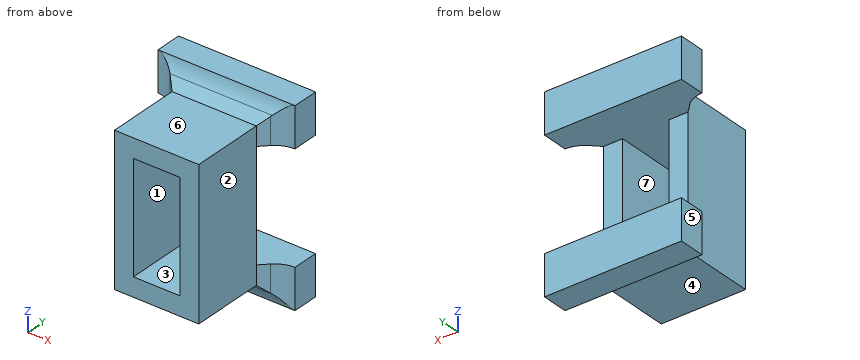
Autodesk Inventor part; units mm, degrees
ref_plane "YZ Plane" through (0, 0, 0) normal (1, 0, 0) x (0, 1, 0)
ref_plane "XZ Plane" through (0, 0, 0) normal (0, 1, 0) x (-1, 0, 0)
ref_plane "XY Plane" through (0, 0, 0) normal (0, 0, 1) x (1, 0, 0)
sketch "Sketch1" plane through (0, 0, 0) normal (0, 1, 0) x (-1, 0, 0)
  line L0 (0, 0) -> (10.16, 0)
  line L1 (10.16, 0) -> (10.16, -17.78)
  line L2 (10.16, -17.78) -> (0, -17.78)
  line L3 (0, -17.78) -> (0, 0)
  line L4 (7.874, -15.494) -> (7.874, -2.286)
  line L5 (7.874, -2.286) -> (2.286, -2.286)
  line L6 (2.286, -2.286) -> (2.286, -15.494)
  line L7 (2.286, -15.494) -> (7.874, -15.494)
  dimension "d0" = 17.78
  dimension "d1" = 10.16
  dimension "d2" = 2.286
extrude "Extrusion1" add sketch "Sketch1" along normal blind 8.89
sketch "Sketch2" plane through (0, 8.89, 0) normal (0, 1, 0) x (1, 0, 0)
  line L0 (-10.16, 0) -> (0, 0)
  line L1 (-2.286, 2.286) -> (-7.874, 2.286)
  line L2 (-7.874, 15.494) -> (-2.286, 15.494)
  line L3 (0, 17.78) -> (-10.16, 17.78)
  line L4 (-10.16, 0) -> (0, 0)
  line L5 (0, 0) -> (0, 2.286)
  line L6 (0, 2.286) -> (-10.16, 2.286)
  line L7 (-10.16, 2.286) -> (-10.16, 0)
  line L8 (-10.16, 0) -> (-10.16, 17.78)
  line L9 (0, 17.78) -> (-10.16, 17.78)
  line L10 (-10.16, 17.78) -> (-10.16, 15.494)
  line L11 (-10.16, 15.494) -> (0, 15.494)
  line L12 (0, 15.494) -> (0, 17.78)
extrude "Extrusion2" add sketch "Sketch2" along normal blind 5.08
sketch "Sketch3" plane through (0, 13.97, 0) normal (0, 1, 0) x (1, 0, 0)
  line L0 (-10.16, 0) -> (0, 0)
  line L1 (0, 17.78) -> (-10.16, 17.78)
  line L2 (-10.16, 15.494) -> (0, 15.494)
  line L3 (0, 15.494) -> (0, 17.78)
  line L4 (0, 17.78) -> (-10.16, 17.78)
  line L5 (-10.16, 17.78) -> (-10.16, 15.494)
  line L6 (-10.16, 0) -> (0, 0)
  line L7 (0, 0) -> (0, 2.286)
  line L8 (0, 2.286) -> (-10.16, 2.286)
  line L9 (-10.16, 2.286) -> (-10.16, 0)
  line L10 (-13.335, 2.286) -> (3.175, 2.286)
  line L11 (3.175, 2.286) -> (3.175, -2.54)
  line L12 (3.175, -2.54) -> (-13.335, -2.54)
  line L13 (-13.335, -2.54) -> (-13.335, 2.286)
  line L14 (-13.335, 15.494) -> (3.175, 15.494)
  line L15 (3.175, 15.494) -> (3.175, 20.32)
  line L16 (3.175, 20.32) -> (-13.335, 20.32)
  line L17 (-13.335, 20.32) -> (-13.335, 15.494)
  dimension "d7" = 3.175
  dimension "d8" = 3.175
  dimension "d9" = 2.54
  dimension "d10" = 2.54
extrude "Extrusion3" add sketch "Sketch3" against normal blind 3.175 contours L0 L7 L10 L11 L12 L13 L9 | L1 L5 L14 L17 L16 L15 L3
chamfer "Chamfer1" distance 1.905 angle 45 6 edges at (-5.08, 10.795, 0) (0, 10.795, -1.143) (-10.16, 10.795, -1.143) (0, 10.795, -16.637) (-5.08, 10.795, -17.78) (-10.16, 10.795, -16.637)
fillet "Fillet1" radius 3.175 6 edges at (1.905, 10.795, -17.5895) (-5.08, 10.795, -19.685) (-12.065, 10.795, -17.5895) (-12.065, 10.795, -0.1905) (-5.08, 10.795, 1.905) (1.905, 10.795, -0.1905)
properties part number "ForeConnectorHolder" material "ABS Plastic"
The model under review builds one solid part; all positions refer to its coordinate system, in mm. Face numbers are marked on the shaded views. A direction names the side the tool comes from. Coordinates: 2 decimals unless noted, no trailing zeros. Order: outer loops, then holes, each group sorted by start corner. A loop starts at its lowest first (then second) coordinate and runs counter-clockwise, first axis right, second up. Notation, with made-up numbers: (63.5, 55) -> (81.5, 55) arc R27 ccw to (81.5, 82) -> close; hole circle Ø10 at (18, 0.5). An arc over 180 degrees is marked (long way). Answer in a Markdown table with one row per item.
(1) Wall thickness on line 1 along X through (y, z) = (5.25, -14); line 2 along Z through (x, y) = (-4.75, 12); line 3 along Z through (x, y) = (-6.5, 3.75): over which ranges is each line inside the solid? List them lowest first.
Answers:
| item | result |
|---|---|
| line 1 | -10.16 to -7.87, -2.29 to 0 |
| line 2 | -20.32 to -15.49, -2.29 to 2.54 |
| line 3 | -17.78 to -15.49, -2.29 to 0 |
(2) Consider section B-B (z = -3.75). Write out the cut boundary in (x, y).
Answers:
| item | result |
|---|---|
| outline | (-10.16, 0) -> (-7.87, 0) -> (-7.87, 8.89) -> (-10.16, 8.89) -> close; (-2.29, 0) -> (0, 0) -> (0, 8.89) -> (-2.29, 8.89) -> close |
(3) The part is to be moulded in two halves that separate along Z. For the marked faces 4, 5, 6 and 7, say which applies: +Z half, -Z half, draft (parallel to the pull), parting line (faces both ways), or undercut.
Answers:
| item | result |
|---|---|
| face 4 | -Z half |
| face 5 | draft |
| face 6 | +Z half |
| face 7 | undercut |
(4) Consider section A-A (y = 9.25). Write out the cut boundary in (x, z).
Answers:
| item | result |
|---|---|
| outline | (-10.52, -18.14) -> (0.36, -18.14) -> (0.36, -15.49) -> (-10.52, -15.49) -> close; (-10.52, -2.29) -> (0.36, -2.29) -> (0.36, 0.36) -> (-10.52, 0.36) -> close |
(5) Machinability: for the marked faces 1, 2 and 3, which of the approach directions +Z, -Z, +X, -X, +Y, -Y give a long, thin tool a straight path to every point of the face, cutting with its end or side? Answer none if there is none.
Answers:
| item | result |
|---|---|
| face 1 | +Y, -Y |
| face 2 | +Z, -Z, +X, -Y |
| face 3 | +Y |
(6) Consider section D-D (z = -18.5). Write out the cut boundary in (x, y) (3 decimals).
Answers:
| item | result |
|---|---|
| outline | (-13.335, 10.795) arc R3.175 cw to (-11.135, 9.865) -> (-10.88, 9.61) -> (0.72, 9.61) -> (0.975, 9.865) arc R3.175 cw to (3.175, 10.795) -> (3.175, 13.97) -> (-13.335, 13.97) -> close |
(7) Insertion check: pin 1 (4 mm diameter, centred on x = -7.5, y = 7, fed in from +Z); pin 2 (2.5 mm diameter, centred on y = 5.5, z = -13, fed in from -X); pin 3 (8 mm diameter, centred on x = -11.5, y = 4, fed in from +Z). Each pin has a flat end and moves straight along its axis. Give the tip position at first contact, or say it passes through.
Answers:
| item | result |
|---|---|
| pin 1 | z = 0.11 |
| pin 2 | x = -10.16 |
| pin 3 | z = 0 |
